from build123d import *

# Parameters (mm, degrees)
SKETCH_1_W             = 13.7
SKETCH_1_H             = 3.7
EXTRUDE_1_DEPTH        = 6.4
CUT_EXTRUDE_1_REACH    = 12.078
EXTRUDE_2_DEPTH        = 0.6
CUT_EXTRUDE_2_REACH    = 16.784
SKETCH_6_W             = 0.5
SKETCH_6_H             = 0.5
CUT_EXTRUDE_3_DEPTH    = 6.05
PATTERN_LINEAR_1_COUNT = 6
PATTERN_LINEAR_1_PITCH = 2
SKETCH_7_W             = 0.5
SKETCH_7_H             = 0.5
CUT_EXTRUDE_4_DEPTH    = 4.5
PATTERN_LINEAR_2_COUNT = 5
PATTERN_LINEAR_2_PITCH = 2
SKETCH_8_W             = 12.5
SKETCH_8_H             = 0.75
CUT_EXTRUDE_5_DEPTH    = 0.75
SKETCH_9_W             = 0.75
SKETCH_9_H             = 3
CUT_EXTRUDE_6_DEPTH    = 0.75
PATTERN_LINEAR_3_COUNT = 7
PATTERN_LINEAR_3_PITCH = 2
SKETCH_10_W            = 0.75
SKETCH_10_H            = 1.264727748
CUT_EXTRUDE_7_DEPTH    = 2.5
PATTERN_LINEAR_4_COUNT = 6
PATTERN_LINEAR_4_PITCH = 2
SKETCH_11_R            = 0.6
CUT_EXTRUDE_8_DEPTH    = 2.5
PATTERN_LINEAR_5_COUNT = 6
PATTERN_LINEAR_5_PITCH = 2
SKETCH_12_R            = 0.45
EXTRUDE_4_DEPTH        = 3
PATTERN_LINEAR_6_COUNT = 6
PATTERN_LINEAR_6_PITCH = 2
SKETCH_15_R            = 0.45
PATTERN_LINEAR_7_COUNT = 6
PATTERN_LINEAR_7_PITCH = 2
SKETCH_16_W            = 19.020248072
SKETCH_16_H            = 7.063508143
CUT_EXTRUDE_9_DEPTH    = 4


with BuildPart() as part:
    # 草图1 → 凸台-拉伸1 (new body)
    with BuildSketch(Plane(origin=(0, 0, 0), x_dir=(1, 0, 0), z_dir=(0, 1, 0))):
        Rectangle(SKETCH_1_W, SKETCH_1_H)
    extrude(amount=EXTRUDE_1_DEPTH)

    # 草图2 → 切除-拉伸1 (cut, up to next)
    with BuildSketch(Plane.XY.offset(1.85), mode=Mode.PRIVATE) as cut_extrude_1_sk1:
        Polygon((-6.25, 0), (-6.25, 6), (-6.85, 6.4), (-6.85, 0), align=None)
    cut_extrude_1_tool1 = extrude(cut_extrude_1_sk1.sketch, amount=-CUT_EXTRUDE_1_REACH, mode=Mode.PRIVATE) & part.part
    # 草图2 → 切除-拉伸1 (cut, up to next)
    with BuildSketch(Plane.XY.offset(1.85), mode=Mode.PRIVATE) as cut_extrude_1_sk2:
        Polygon((6.85, 0), (6.25, 0), (6.25, 6), (6.85, 6.4), align=None)
    cut_extrude_1_tool2 = extrude(cut_extrude_1_sk2.sketch, amount=-CUT_EXTRUDE_1_REACH, mode=Mode.PRIVATE) & part.part
    add(cut_extrude_1_tool1.solids().sort_by_distance((-6.553226, 3.101075, 1.85))[0], mode=Mode.SUBTRACT)
    add(cut_extrude_1_tool2.solids().sort_by_distance((6.553226, 3.101075, 1.85))[0], mode=Mode.SUBTRACT)

    # 草图4 → 凸台-拉伸2 (add)
    with BuildSketch(Plane.XY.offset(1.85)):
        Polygon((-3.65, 0), (-2.875, 0), (-2.875, 5.4), (2.875, 5.4), (2.875, 0), (3.65, 0), (3.65, 6.4), (-3.65, 6.4), align=None)
    extrude(amount=EXTRUDE_2_DEPTH)

    # 切除-拉伸2: up to this face of the body (flat: up to its plane)
    cut_extrude_2_end = Plane(part.part.faces().sort_by_distance((6.25, 3, 0))[0])
    # 草图5 → 切除-拉伸2 (cut, up to the picked face)
    with BuildSketch(Plane.ZY.offset(6.25), mode=Mode.PRIVATE) as cut_extrude_2_sk1:
        Polygon((2.45, 0.35), (0.45, 0.35), (0, 0), (2.45, 0), align=None)
    cut_extrude_2_tool1 = split(extrude(cut_extrude_2_sk1.sketch, amount=-CUT_EXTRUDE_2_REACH, mode=Mode.PRIVATE), bisect_by=cut_extrude_2_end, keep=Keep.BOTH, mode=Mode.PRIVATE)
    add(cut_extrude_2_tool1.solids().sort_by(Axis((-6.25, 0.169101, 1.333708), (1, 0, 0)))[0], mode=Mode.SUBTRACT)

    # 草图6 → 切除-拉伸3 (cut)
    with BuildSketch(Plane.XZ.offset(-0.35)):
        with Locations((-5, 0.7)):
            Rectangle(SKETCH_6_W, SKETCH_6_H)
    cut_extrude_3 = extrude(amount=-CUT_EXTRUDE_3_DEPTH, mode=Mode.SUBTRACT)

    # 阵列(线性)1: 切除-拉伸3 ×6
    with Locations(*[(i * PATTERN_LINEAR_1_PITCH, 0, 0) for i in range(1, PATTERN_LINEAR_1_COUNT)]):
        add(cut_extrude_3, mode=Mode.SUBTRACT)

    # 草图7 → 切除-拉伸4 (cut)
    with BuildSketch(Plane.XZ):
        with Locations((-4, -1.6)):
            Rectangle(SKETCH_7_W, SKETCH_7_H)
    cut_extrude_4 = extrude(amount=-CUT_EXTRUDE_4_DEPTH, mode=Mode.SUBTRACT)

    # 阵列(线性)2: 切除-拉伸4 ×5
    with Locations(*[(i * PATTERN_LINEAR_2_PITCH, 0, 0) for i in range(1, PATTERN_LINEAR_2_COUNT)]):
        add(cut_extrude_4, mode=Mode.SUBTRACT)

    # 草图8 → 切除-拉伸5 (cut)
    with BuildSketch(Plane(origin=(0, 0, -1.85), x_dir=(-1, 0, 0), z_dir=(0, 0, -1))):
        with Locations((0, 1.875)):
            Rectangle(SKETCH_8_W, SKETCH_8_H)
    extrude(amount=-CUT_EXTRUDE_5_DEPTH, mode=Mode.SUBTRACT)

    # 草图9 → 切除-拉伸6 (cut)
    with BuildSketch(Plane(origin=(0, 0, -1.85), x_dir=(-1, 0, 0), z_dir=(0, 0, -1))):
        with Locations((-6, 3)):
            Rectangle(SKETCH_9_W, SKETCH_9_H)
    cut_extrude_6 = extrude(amount=-CUT_EXTRUDE_6_DEPTH, mode=Mode.SUBTRACT)

    # 阵列(线性)3: 切除-拉伸6 ×7
    with Locations(*[(-i * PATTERN_LINEAR_3_PITCH, 0, 0) for i in range(1, PATTERN_LINEAR_3_COUNT)]):
        add(cut_extrude_6, mode=Mode.SUBTRACT)

    # 草图10 → 切除-拉伸7 (cut)
    with BuildSketch(Plane(origin=(0, 0, -1.85), x_dir=(-1, 0, 0), z_dir=(0, 0, -1))):
        with Locations((-5, 1.232363874)):
            Rectangle(SKETCH_10_W, SKETCH_10_H)
    cut_extrude_7 = extrude(amount=-CUT_EXTRUDE_7_DEPTH, mode=Mode.SUBTRACT)

    # 阵列(线性)4: 切除-拉伸7 ×6
    with Locations(*[(-i * PATTERN_LINEAR_4_PITCH, 0, 0) for i in range(1, PATTERN_LINEAR_4_COUNT)]):
        add(cut_extrude_7, mode=Mode.SUBTRACT)

    # 草图11 → 切除-拉伸8 (cut)
    with BuildSketch(Plane(origin=(0, 6.4, 0), x_dir=(1, 0, 0), z_dir=(0, 1, 0))):
        with Locations((-5, 0)):
            Circle(SKETCH_11_R)
    cut_extrude_8 = extrude(amount=-CUT_EXTRUDE_8_DEPTH, mode=Mode.SUBTRACT)

    # 阵列(线性)5: 切除-拉伸8 ×6
    with Locations(*[(i * PATTERN_LINEAR_5_PITCH, 0, 0) for i in range(1, PATTERN_LINEAR_5_COUNT)]):
        add(cut_extrude_8, mode=Mode.SUBTRACT)

    # 草图12 → 凸台-拉伸4 (add)
    with BuildSketch(Plane(origin=(0, 3.9, 0), x_dir=(1, 0, 0), z_dir=(0, 1, 0))):
        with Locations(Location((-5, 0, 0), (0, 0, 270))):
            Circle(SKETCH_12_R)
    extrude_4 = extrude(amount=EXTRUDE_4_DEPTH)

    # 阵列(线性)6: 凸台-拉伸4 ×6
    with Locations(*[(i * PATTERN_LINEAR_6_PITCH, 0, 0) for i in range(1, PATTERN_LINEAR_6_COUNT)]):
        add(extrude_4)

    # 扫描1: sweep along a path in 草图13
    with BuildLine(Plane.ZY.offset(5)) as sweep_1_path:
        Line((0, 6.9), (0, 13.072800135))
    # 草图15 → 扫描1 (sweep)
    with BuildSketch(Plane(origin=(0, 6.9, 0), x_dir=(1, 0, 0), z_dir=(0, 1, 0))):
        with Locations((-5, 0)):
            Circle(SKETCH_15_R)
    sweep_1 = sweep(path=sweep_1_path.line)

    # 阵列(线性)7: 扫描1 ×6
    with Locations(*[(i * PATTERN_LINEAR_7_PITCH, 0, 0) for i in range(1, PATTERN_LINEAR_7_COUNT)]):
        add(sweep_1)

    # 草图16 → 切除-拉伸9 (cut)
    with BuildSketch(Plane(origin=(0, 13.072800135, 0), x_dir=(1, 0, 0), z_dir=(0, 1, 0))):
        with Locations((-1.031218269, 0.439526414)):
            Rectangle(SKETCH_16_W, SKETCH_16_H)
    extrude(amount=-CUT_EXTRUDE_9_DEPTH, mode=Mode.SUBTRACT)


solid = part.part
Work out the finished part from the listing and answer in its coordinate system (mm). A direction names the side the tool comes from. Give positions to 0.01 mm unless a question says otherwise; leave off trailing zeros. Loops run counter-clockwise (first coordinate to the right, second up) from the corner with the lowest first, then second, coordinate; pieces in that order, holes last. Notation, with made-up numbers: (7.25, -34.75) -> (40.25, -34.75) arc R17 ccw to (40.25, -25.75) -> close; hole circle Ø4 at (-21, -37.5). An arc over 180 degrees is marked (long way). Use a Markdown table: item, result. Add a question column.
1) The part is cut by section B-B, the plane z = 1.45. Determine the outline of the cut face in (x, y), plus the area to 3 significant figures.
2) Each of these flat-tipped pins is pushed along its axis until it touches: P1, Ø1.6, axis at x = 5, y = 2, coming from the +Z side; P2, Ø4, axis at x = 5.5, y = 6.5, coming from the -Z side. Where does it stop, or does it pass through?
3) Which of the six approach directions +Z, -Z, +X, -X, +Y, -Y give full straight-line access (tool end or side, diameter ignored) to faces 4 (the flat face through (0.625, 1, -1)), 5 (the flat face through (5, 3, 1.85)), 6 (the flat face through (6.25, 3, 0))?
4) Consider line 1 along X through (y, z) = (7.75, 0.15); line 2 along Y through (x, z) = (5, -1.15); line 3 along Y through (x, z) = (0.75, -0.7). Determine where each line is inside the solid, lowest interval first.
5) The part is cut by section A-A, the plane y = 7.5. Determine the outline of the cut face in (x, z), plus the area to 3 significant figures.
6) For a pull along Z with two mould halves and no side action, classify faces 1 (the flat face through (3, 0.4, -1.85)), 2 (the flat face through (0, 3, 1.85)), 3 (the cylindrical face through (-4.98, 5.17, -0.6)) as +Z half, -Z half, draft (parallel to the pull), parting line (faces both ways), or undercut.
7) The part is cut by section C-C, the plane z = 0.2. Count the separate pieces of the cut face and the enclosed holes in it, plus the area to 3 significant figures.
Reported:
| question | item | result |
|---|---|---|
| 1 | outline | (-6.85, 6.4) -> (-6.25, 6) -> (-6.25, 0.35) -> (6.25, 0.35) -> (6.25, 6) -> (6.85, 6.4) -> close |
| 1 | area | 75.9 mm^2 |
| 2 | P1 | stops at z = 1.85 |
| 2 | P2 | stops at z = -1.85 |
| 3 | face 4 | -Z |
| 3 | face 5 | +Z, +X, +Y, -Y |
| 3 | face 6 | +Z, -Z, +X, -Y |
| 4 | line 1 | x = -5.42 to -4.58, -3.42 to -2.58, -1.42 to -0.58, 0.58 to 1.42, 2.58 to 3.42, 4.58 to 5.42 |
| 4 | line 2 | y = 0 to 0.6, 2.25 to 6.4 |
| 4 | line 3 | y = 0 to 0.6, 1.86 to 6.4 |
| 5 | outline | circle Ø0.9 at (-5, 0); circle Ø0.9 at (-3, 0); circle Ø0.9 at (-1, 0); circle Ø0.9 at (1, 0); circle Ø0.9 at (3, 0); circle Ø0.9 at (5, 0) |
| 5 | area | 3.82 mm^2 |
| 6 | face 1 | -Z half |
| 6 | face 2 | +Z half |
| 6 | face 3 | undercut |
| 7 | separate pieces | 1 |
| 7 | enclosed holes | 6 |
| 7 | area | 80.7 mm^2 |
